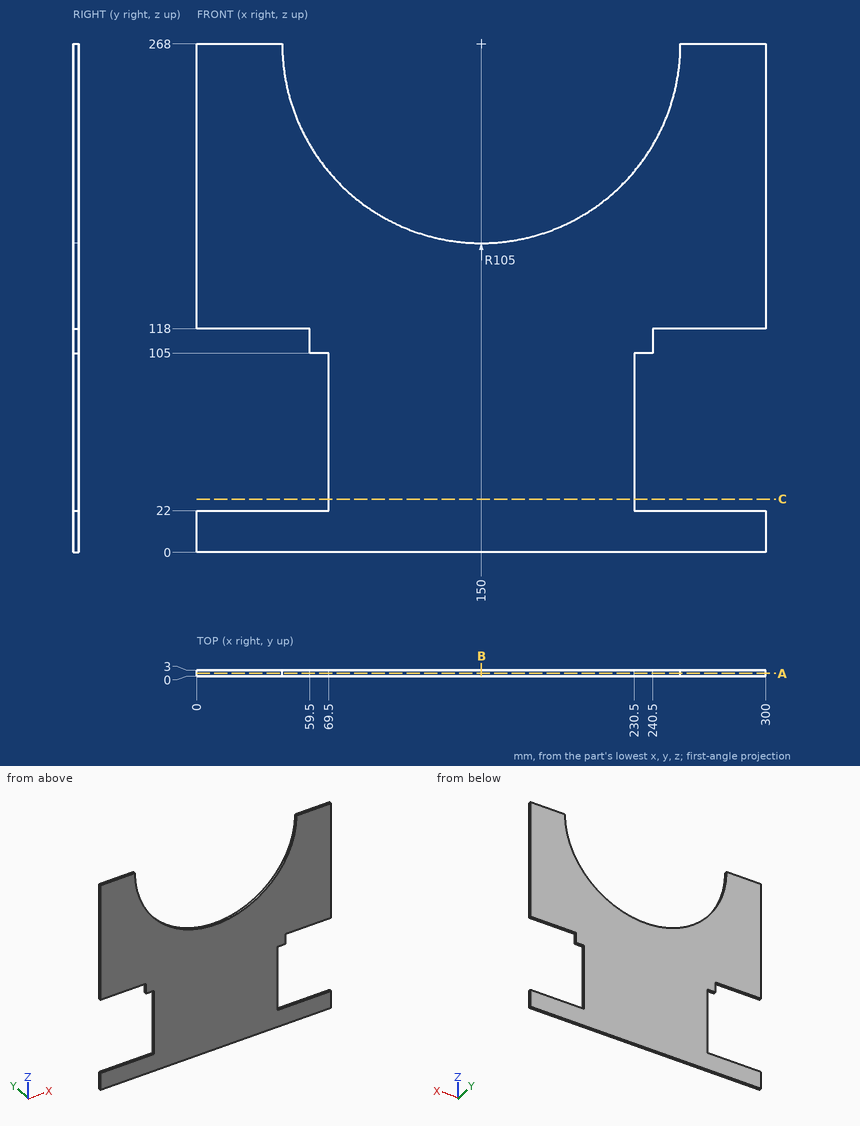
Geometry check sheet. Reference: drawing and pictorial views, mm from the part's lowest x, y, z. Coordinates: 2 decimals unless noted, no trailing zeros. Order: outer loops, then holes, each group sorted by start corner. A loop starts at its lowest first (then second) coordinate and runs counter-clockwise, first axis right, second up.
1. Sectioned sample at C-C, the plane z = 28. Record the cut outline in (x, y).
Results found:
outline: (69.5, 0) - (230.5, 0) - (230.5, 3) - (69.5, 3) - close
2. Sectioned sample at A-A, the plane y = 1.4. Record the cut outline in (x, z).
Results found:
outline: (0, 0) - (300, 0) - (300, 22) - (230.5, 22) - (230.5, 105) - (240.5, 105) - (240.5, 118) - (300, 118) - (300, 268) - (255, 268) arc R105 cw to (45, 268) - (0, 268) - (0, 118) - (59.5, 118) - (59.5, 105) - (69.5, 105) - (69.5, 22) - (0, 22) - close
3. Go/stop test with flat-tipped pins: pin 1 Ø0.9 at (y, z) = (1, 43.5) entering from +X; pin 2 Ø1.5 at (y, z) = (2, 109.5) entering from +X. Record where each tip stops, or that it passes through.
Results found:
pin 1: stops at x = 230.5
pin 2: stops at x = 240.5
4. Sectioned sample at B-B, the plane x = 150. Record the cut outline in (y, z).
Results found:
outline: (0, 0) - (3, 0) - (3, 163) - (0, 163) - close
5. Scan lines: line 1 (Z direction, x = 272, y = 0.45); line 2 (X direction, y = 1.85, z = 76); line 3 (Z direction, x = 233, y = 0.45). Record each from-to range of solid material in increasing order.
Results found:
line 1: z = 0 to 22, 118 to 268
line 2: x = 69.5 to 230.5
line 3: z = 0 to 22, 105 to 203.69
